Build history of the part. All positions in model axes, mm. Face numbers are marked on the shaded views. A direction names the side the tool comes from. Round coordinates to 2 decimals unless told otherwise and drop trailing zeros. Loops run counter-clockwise (first coordinate to the right, second up) from the corner with the lowest first, then second, coordinate; pieces in that order, holes last. Notation, with made-up numbers: (10, 41) -> (68, 41) arc R26 cw to (68, 80) -> close; hole circle Ø8 at (3.5, 43). An arc over 180 degrees is marked (long way). Put each result on its own line as item: value. Start each with the question number.
Item 1: Cut at B-B, the plane y = -4.75. List the corners of the cut face in (x, z).
Item 2: Drill centre lines: probe 1 along X at (y, z) = (-2.15, 0); probe 2 along Z at (x, y) = (0, -1.9); probe 3 along X at (y, z) = (-4.1, 0). Where is each one in solid material? Low to high. Write a range as [from, to].
Item 3: Flat gauge pin, fed straight in: pin 1 Ø2 at (y, z) = (-3, 3) entering from +X. Where does the tip first touch, or does it go through?
Item 4: Tool access for the marked faces 1, 2, 3, 4 and 5: list every direction of +Z, -Z, +X, -X, +Y, -Y with a clear straight run to the whole face (end or side of a thin tool).
Item 5: Cut at A-A, the plane y = -2.5. List the corners of the cut face in (x, z), plus the area to 3 significant figures.
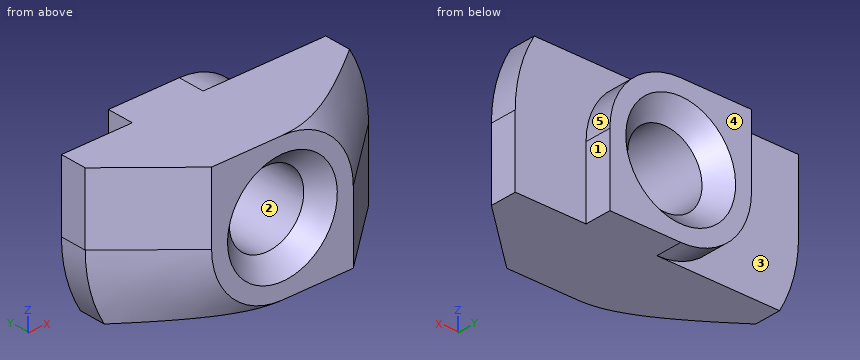
```python
from build123d import *

# Parameters (mm, degrees)
EXTRUDE_1_DEPTH     = 4
CUT_EXTRUDE_1_DEPTH = 1.5
CUT_EXTRUDE_2_DEPTH = 6


with BuildPart() as part:
    # Эскиз1 → Бобышка-Вытянуть1 (new body, symmetric)
    with BuildSketch(Plane.XY):
        Polygon((4, 0), (-4, 0), (-4, -1.5), (-8, -1.5), (-8, -6.5), (8, -6.5), (8, -1.5), (4, -1.5), align=None)
    extrude(amount=EXTRUDE_1_DEPTH, both=True)

    # Эскиз3 → Отверстие обработанное метчиком M52 (revolve, cut)
    with BuildSketch(Plane(origin=(0, 0, 0), x_dir=(0, 0, 1), z_dir=(1, 0, 0))):
        Polygon((0, 0), (0, 6.5), (3.1, 6.5), (2.1, 5.5), (2.1, 1), (3.1, 0), align=None)
    revolve(axis=Axis((0, 6.35, 0), (0, -1, 0)), mode=Mode.SUBTRACT)

    # Эскиз4 → Вырез-Вытянуть1 (cut)
    with BuildSketch(Plane(origin=(0, 0, 0), x_dir=(1, 0, 0), z_dir=(0, 1, 0))):
        with BuildLine():
            Line((-4, 4), (-4, 0))
            ThreePointArc((-4, 0), (-2.828427125, 2.828427125), (0, 4))
            Line((0, 4), (-4, 4))
        make_face()
        with BuildLine():
            Line((0, -4), (4, -4))
            Line((4, -4), (4, 0))
            ThreePointArc((4, 0), (2.828427125, -2.828427125), (0, -4))
        make_face()
    extrude(amount=-CUT_EXTRUDE_1_DEPTH, mode=Mode.SUBTRACT)

    # Эскиз5 → Вырез-Вытянуть2 (cut, through all)
    with BuildSketch(Plane(origin=(0, -1.5, 0), x_dir=(1, 0, 0), z_dir=(0, 1, 0))):
        with BuildLine():
            Line((-8, 0), (-8, 4))
            Line((-8, 4), (-6.92820323, 4))
            ThreePointArc((-6.92820323, 4), (-7.72740661, 2.070552361), (-8, 0))
        make_face()
        with BuildLine():
            Line((8, 0), (8, -4))
            Line((8, -4), (6.92820323, -4))
            ThreePointArc((6.92820323, -4), (7.72740661, -2.070552361), (8, 0))
        make_face()
    extrude(amount=-CUT_EXTRUDE_2_DEPTH, mode=Mode.SUBTRACT)

    # Вырез-По траектории1: sweep along a path in Эскиз7
    with BuildLine(Plane.XZ.offset(6.5)) as sweep_1_path:
        Line((0, 8), (-8, 8))
        Line((-8, 8), (-8, 0))
        ThreePointArc((-8, 0), (-5.656854249, -5.656854249), (0, -8))
        Line((0, -8), (8, -8))
        Line((8, -8), (8, 0))
        ThreePointArc((8, 0), (5.656854249, 5.656854249), (0, 8))
    # Эскиз6 → Вырез-По траектории1 (sweep, cut)
    with BuildSketch(Plane.XY.offset(4)):
        Polygon((-8, -3), (-8, -6.5), (-4, -6.5), align=None)
    sweep(path=sweep_1_path.line, transition=Transition.RIGHT, mode=Mode.SUBTRACT)


solid = part.part
```
Reply:
1. outline: (-6, 0) arc R6 ccw to (-4.47, -4) -> (6, -4) -> (6, 0) arc R6 ccw to (4.47, 4) -> (-6, 4) -> close; hole circle Ø4.2 at (0, 0)
2. probe 1: x = [-8, -2.1], [2.1, 8]
2. probe 2: z = [-4, -2.1], [2.1, 4]
2. probe 3: x = [-6.74, -2.1], [2.1, 6.74]
3. pin 1: stops at x = 7.75
4. face 1: +Z, -Z, +X, +Y
4. face 2: +Y, -Y
4. face 3: -Z, -X, +Y
4. face 4: +Z, -Z, +X, -X, +Y
4. face 5: +Z, +X, +Y
5. outline: (-8, 0) arc R8 ccw to (-6.93, -4) -> (8, -4) -> (8, 0) arc R8 ccw to (6.93, 4) -> (-8, 4) -> close; hole circle Ø4.2 at (0, 0)
5. area: 111 mm^2
